Input: part model. Units: mm. Frame: model coordinates. Face numbers are marked on the shaded views. A direction names the side the tool comes from. Round coordinates to 2 decimals unless told otherwise and drop trailing zeros. Loops run counter-clockwise (first coordinate to the right, second up) from the corner with the lowest first, then second, coordinate; pieces in that order, holes last.
(1) Line query: line 1 (Z direction, x = -2, y = 32); line 2 (Y direction, x = -1.25, z = -39); line 3 (Z direction, x = 105.5, y = -5.5). Output: solid intervals per line, ascending.
(2) Cut plane A-A, the plane z = -6.5. Output: boundary loops of the cut face in (x, y), and give its area (3 significant figures).
(3) Access query for the marked faces 3 and 4. Directions: +Z, -Z, +X, -X, +Y, -Y. A direction counts if a zero-diameter tool reaches every point of the face in a straight line with its end or side. Return the directions, or none.
(4) First-contact query: pin 1 Ø4 at (x, z) = (8.5, -22.5) entering from +Y; pin 2 Ø12 at (y, z) = (0.5, -47.5) entering from +X; pin 3 Ø10 at (x, y) = (12.5, 2) entering from -Z. Flat tips, straight axial feed; report the tip coordinate or a pass-through.
(5) Cut plane C-C, the plane z = -22.75. Output: boundary loops of the cut face in (x, y), and give its area (3 significant figures).
(6) Cut plane D-D, the plane y = 3.5. Output: boundary loops of the cut face in (x, z).
(7) Cut plane B-B, the plane y = 32.5. Output: boundary loops of the cut face in (x, z), and give its area (4 significant figures).
(8) Draft query along X for the marked faces 1 and 2. Return one class per face: released by +X, released by -X, zero draft, split by the parting line, or undercut.
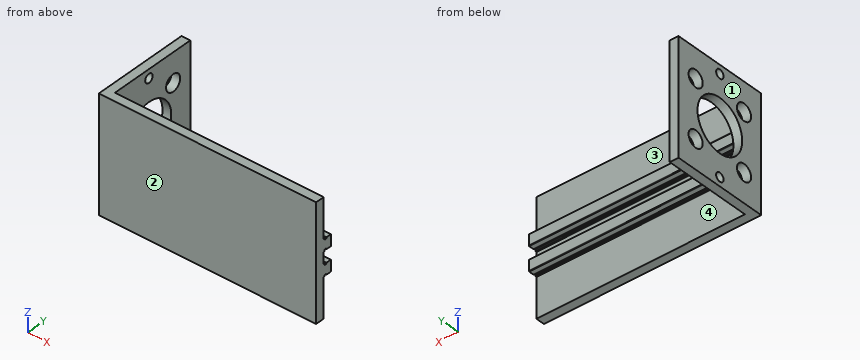
Autodesk Inventor part; units mm, degrees
ref_plane "YZ Plane" through (0, 0, 0) normal (1, 0, 0) x (0, 1, 0)
ref_plane "XZ Plane" through (0, 0, 0) normal (0, 1, 0) x (-1, 0, 0)
ref_plane "XY Plane" through (0, 0, 0) normal (0, 0, 1) x (1, 0, 0)
sketch "Sketch4" plane through (0, 0, 0) normal (1, 0, 0) x (0, 1, 0)
  line L0 (-6, -12.5) -> (-6, -12.9)
  arc A0 (-6, -12.9) -> (-5.6, -13.3) centre (-5.6, -12.9) ccw
  line L1 (-5.6, -13.3) -> (-4.9, -13.3)
  arc A1 (-4.9, -13.3) -> (-4.7, -13.1) centre (-4.9, -13.1) ccw
  line L2 (-4.7, -13.1) -> (-4.7, -12.85)
  arc A2 (-4.5, -12.65) -> (-4.7, -12.85) centre (-4.5, -12.85) ccw
  line L3 (-4.5, -12.65) -> (-1.8, -12.65)
  arc A3 (-1.4, -13.05) -> (-1.8, -12.65) centre (-1.8, -13.05) ccw
  line L4 (-1.4, -13.05) -> (-1.4, -18.75)
  line L5 (-1.8, -19.15) -> (-4.5, -19.15)
  arc A4 (-1.8, -19.15) -> (-1.4, -18.75) centre (-1.8, -18.75) ccw
  arc A5 (-4.7, -18.95) -> (-4.5, -19.15) centre (-4.5, -18.95) ccw
  line L6 (-4.7, -18.95) -> (-4.7, -18.7)
  arc A6 (-4.7, -18.7) -> (-4.9, -18.5) centre (-4.9, -18.7) ccw
  line L7 (-4.9, -18.5) -> (-5.6, -18.5)
  arc A7 (-5.6, -18.5) -> (-6, -18.9) centre (-5.6, -18.9) ccw
  line L8 (-6, -18.9) -> (-6, -19.5)
  line L9 (-6.5, -6.5) -> (-6.5, -12.5)
  line L10 (-6.5, -12.5) -> (-6, -12.5)
  line L11 (-6, -19.5) -> (-6.5, -19.5)
  line L12 (-6.5, -19.5) -> (-6.5, -26)
  line L13 (-6.5, -26) -> (-6, -26)
  line L14 (-6, -26) -> (-6, -26.6)
  arc A8 (-6, -26.6) -> (-5.6, -27) centre (-5.6, -26.6) ccw
  line L15 (-5.6, -27) -> (-4.9, -27)
  arc A9 (-4.9, -27) -> (-4.7, -26.8) centre (-4.9, -26.8) ccw
  arc A10 (-4.5, -26.35) -> (-4.7, -26.55) centre (-4.5, -26.55) ccw
  line L16 (-4.7, -26.8) -> (-4.7, -26.55)
  line L17 (-4.5, -26.35) -> (-1.8, -26.35)
  arc A11 (-1.4, -26.75) -> (-1.8, -26.35) centre (-1.8, -26.75) ccw
  line L18 (-1.4, -26.75) -> (-1.4, -32.45)
  arc A12 (-1.8, -32.85) -> (-1.4, -32.45) centre (-1.8, -32.45) ccw
  line L19 (-1.8, -32.85) -> (-4.5, -32.85)
  arc A13 (-4.7, -32.65) -> (-4.5, -32.85) centre (-4.5, -32.65) ccw
  line L20 (-4.7, -32.65) -> (-4.7, -32.4)
  arc A14 (-4.7, -32.4) -> (-4.9, -32.2) centre (-4.9, -32.4) ccw
  line L21 (-4.9, -32.2) -> (-5.6, -32.2)
  arc A15 (-5.6, -32.2) -> (-6, -32.6) centre (-5.6, -32.6) ccw
  line L22 (-6, -32.6) -> (-6, -33)
  line L23 (-6, -33) -> (-6.5, -33)
  line L24 (-6.5, -33) -> (-6.5, -39)
  circle A16 centre (0, -6.5) radius 4.75
  circle A17 centre (32.5, -6.5) radius 4.75
  circle A18 centre (0, -39) radius 4.75
  circle A19 centre (32.5, -39) radius 4.75
  line L25 (39, -26) -> (39, -19.5)
  line L26 (39, -12.5) -> (39, -6.5)
  line L27 (39, -39) -> (39, -33)
  line L28 (39, -45.5) -> (39, 0)
  line L29 (39, -45.5) -> (39, -55.5)
  line L30 (39, -55.5) -> (-6.5, -55.5)
  line L31 (-6.5, -55.5) -> (-6.5, -45.5)
  line L32 (39, 0) -> (39, 10)
  line L33 (39, 10) -> (-6.5, 10)
  line L34 (-6.5, 10) -> (-6.5, 0)
  line L35 (-6.5, 0) -> (-6.5, -12.5)
  line L36 (-6.5, -19.5) -> (-6.5, -26)
  line L37 (-6.5, -33) -> (-6.5, -45.5)
  line L38 (-6.5, 10) -> (-11.5, 10)
  line L39 (-11.5, 10) -> (-11.5, -55.5)
  line L40 (-11.5, -55.5) -> (-6.5, -55.5)
  line L41 (-6.5, -12.5) -> (-6.5, 10)
  line L42 (-6.5, -55.5) -> (-6.5, -33)
  line L43 (-6.5, -26) -> (-6.5, -19.5)
  point P0 (0, 0)
  dimension "d36" = 10
  dimension "d37" = 10
  dimension "d38" = 5
extrude "Extrusion6" add sketch "Sketch4" along normal blind 118.9 contours L0 A0 L1 A1 L2 A2 L3 A3 L4 A4 L5 A5 L6 A6 L7 A7 L8 L11 L12 L13 L14 A8 L15 A9 L16 A10 L17 A11 L18 A12 L19 A13 L20 A14 L21 A15 L22 L23 L24 L37 L31 L40 L39 L38 L34 L35 L9 L10
sketch "Sketch5" plane through (0, 0, 0) normal (-1, 0, 0) x (0, 0, 1)
  line L0 (-33, -6) -> (-32.6, -6)
  arc A0 (-32.6, -6) -> (-32.2, -5.6) centre (-32.6, -5.6) ccw
  line L1 (-32.2, -5.6) -> (-32.2, -4.9)
  arc A1 (-32.2, -4.9) -> (-32.4, -4.7) centre (-32.4, -4.9) ccw
  line L2 (-32.4, -4.7) -> (-32.65, -4.7)
  arc A2 (-32.85, -4.5) -> (-32.65, -4.7) centre (-32.65, -4.5) ccw
  line L3 (-32.85, -4.5) -> (-32.85, -1.8)
  arc A3 (-32.45, -1.4) -> (-32.85, -1.8) centre (-32.45, -1.8) ccw
  line L4 (-32.45, -1.4) -> (-26.75, -1.4)
  line L5 (-26.35, -1.8) -> (-26.35, -4.5)
  arc A4 (-26.35, -1.8) -> (-26.75, -1.4) centre (-26.75, -1.8) ccw
  arc A5 (-26.55, -4.7) -> (-26.35, -4.5) centre (-26.55, -4.5) ccw
  line L6 (-26.55, -4.7) -> (-26.8, -4.7)
  arc A6 (-26.8, -4.7) -> (-27, -4.9) centre (-26.8, -4.9) ccw
  line L7 (-27, -4.9) -> (-27, -5.6)
  arc A7 (-27, -5.6) -> (-26.6, -6) centre (-26.6, -5.6) ccw
  line L8 (-26.6, -6) -> (-26, -6)
  line L9 (-39, -6.5) -> (-33, -6.5)
  line L10 (-33, -6.5) -> (-33, -2.5)
  line L11 (-26, -1.05) -> (-26, -6.5)
  line L12 (-26, -6.5) -> (-19.5, -6.5)
  line L13 (-19.5, -6.5) -> (-19.5, -1.05)
  line L14 (-19.5, -6) -> (-18.9, -6)
  arc A8 (-18.9, -6) -> (-18.5, -5.6) centre (-18.9, -5.6) ccw
  line L15 (-18.5, -5.6) -> (-18.5, -4.9)
  arc A9 (-18.5, -4.9) -> (-18.7, -4.7) centre (-18.7, -4.9) ccw
  arc A10 (-19.15, -4.5) -> (-18.95, -4.7) centre (-18.95, -4.5) ccw
  line L16 (-18.7, -4.7) -> (-18.95, -4.7)
  line L17 (-19.15, -4.5) -> (-19.15, -1.8)
  arc A11 (-18.75, -1.4) -> (-19.15, -1.8) centre (-18.75, -1.8) ccw
  line L18 (-18.75, -1.4) -> (-13.05, -1.4)
  arc A12 (-12.65, -1.8) -> (-13.05, -1.4) centre (-13.05, -1.8) ccw
  line L19 (-12.65, -1.8) -> (-12.65, -4.5)
  arc A13 (-12.85, -4.7) -> (-12.65, -4.5) centre (-12.85, -4.5) ccw
  line L20 (-12.85, -4.7) -> (-13.1, -4.7)
  arc A14 (-13.1, -4.7) -> (-13.3, -4.9) centre (-13.1, -4.9) ccw
  line L21 (-13.3, -4.9) -> (-13.3, -5.6)
  arc A15 (-13.3, -5.6) -> (-12.9, -6) centre (-12.9, -5.6) ccw
  line L22 (-12.9, -6) -> (-12.5, -6)
  line L23 (-12.5, -2.5) -> (-12.5, -6.5)
  line L24 (-12.5, -6.5) -> (-6.5, -6.5)
  line L25 (-45.5, 32.5) -> (-45.5, 0)
  circle A16 centre (-39, 0) radius 4.75
  circle A17 centre (-39, 32.5) radius 4.75
  circle A18 centre (-6.5, 0) radius 4.75
  circle A19 centre (-6.5, 32.5) radius 4.75
  line L26 (-19.5, 39) -> (-26, 39)
  line L27 (-33, 39) -> (-39, 39)
  line L28 (-6.5, 39) -> (-12.5, 39)
  line L29 (0, 26.5) -> (0, 32.5)
  line L30 (0, 0) -> (0, 6)
  line L31 (0, 13) -> (0, 19.5)
  circle A20 centre (-22.75, 16.25) radius 15
  line L32 (-12.5, -6) -> (-12.5, -6.5)
  line L33 (10, -11.5) -> (-55.5, -11.5)
  line L34 (10, -11.5) -> (-55.5, -11.5)
  line L35 (-55.5, -11.5) -> (-55.5, 44)
  line L36 (-55.5, 44) -> (10, 44)
  line L37 (10, 44) -> (10, -11.5)
  line L38 (10, 39) -> (10, 44)
  point P0 (0, 0)
  point P1 (-55.5, -11.5)
  dimension "d43" = 5
extrude "Extrusion7" add sketch "Sketch5" along normal blind 5
sketch "Sketch7" plane through (-5, 0, 0) normal (-1, 0, 0) x (0, 0, 1)
  line L0 (10, -11.5) -> (10, 44)
  line L1 (10, 44) -> (0, -11.5)
  line L2 (-55.5, -11.5) -> (10, -11.5)
  line L3 (10, -11.5) -> (0, 44)
  line L4 (10, 44) -> (-55.5, 44)
  line L5 (-55.5, 44) -> (-55.5, -11.5)
  line L6 (-55.5, -10.3017) -> (-45.7159, 44)
  line L7 (-45.7159, 44) -> (-55.5, 44)
  line L8 (-55.5, 44) -> (-45.5032, -11.4823)
  circle A0 centre (5, 16.25) radius 2.5
  circle A1 centre (-50.5016, 16.2588) radius 2.5
  point P0 (0, 0)
  dimension "d44" = 5
  dimension "d45" = 5
extrude "Extrusion8" cut sketch "Sketch7" against normal through all contours A0 L1 L3 | L3 L1 A0 | L1 L3 A0 | A0 L3 L1 | A1 L8 L6 | L6 L8 A1 | A1 L8 L6 | L6 L8 A1
properties part number "SoporteHidráhulicos_CPY" material "Steel, Mild, Welded"
Reported:
1. line 1: z = -55.5 to -43.72, -34.28 to -11.22, -1.78 to 10
1. line 2: y = -11.5 to -4.75, 4.75 to 27.75, 37.25 to 44
1. line 3: z = -32.2 to -27, -18.5 to -13.3
2. outline: (-5, -11.5) - (118.9, -11.5) - (118.9, -6.5) - (0, -6.5) - (0, -4.75) - (-5, -4.75) - close; (-5, 4.75) - (0, 4.75) - (0, 27.75) - (-5, 27.75) - close; (-5, 37.25) - (0, 37.25) - (0, 44) - (-5, 44) - close
2. area: 777 mm2
3. face 3: +Z, +X, +Y
3. face 4: -Z, +X, +Y
4. pin 1: stops at y = -6.5
4. pin 2: stops at x = 0
4. pin 3: stops at z = -32.85
5. outline: (-5, -11.5) - (118.9, -11.5) - (118.9, -6.5) - (0, -6.5) - (0, 1.25) - (-5, 1.25) - close; (-5, 31.25) - (0, 31.25) - (0, 44) - (-5, 44) - close
5. area: 722 mm2
6. outline: (-5, -55.5) - (0, -55.5) - (0, -42.21) - (-5, -42.21) - close; (-5, -35.79) - (0, -35.79) - (0, -30.65) - (-5, -30.65) - close; (-5, -14.85) - (0, -14.85) - (0, -9.71) - (-5, -9.71) - close; (-5, -3.29) - (0, -3.29) - (0, 10) - (-5, 10) - close
7. outline: (-5, -55.5) - (0, -55.5) - (0, -43.75) - (-5, -43.75) - close; (-5, -34.25) - (0, -34.25) - (0, -11.25) - (-5, -11.25) - close; (-5, -1.75) - (0, -1.75) - (0, 10) - (-5, 10) - close
7. area: 232.5 mm2
8. face 1: released by -X
8. face 2: zero draft
